from build123d import *

# Parameters (mm, degrees)
SKETCH_1_R          = 21
EXTRUDE_1_DEPTH     = 67
SKETCH_3_R          = 7.5
EXTRUDE_3_DEPTH     = 4.5
SKETCH_4_R          = 2.5
EXTRUDE_4_DEPTH     = 12.7
FILLET_1_R          = 2
FILLET_2_R          = 1
SKETCH_15_R         = 2
CUT_EXTRUDE_2_DEPTH = 5
SKETCH_18_W         = 4.6
SKETCH_18_H         = 0.6
EXTRUDE_11_DEPTH    = 7
SKETCH_19_R         = 7.6
EXTRUDE_12_DEPTH    = 7
EXTRUDE_START       = -39.2
SKETCH_20_R         = 22.175
SKETCH_20_R_2       = 21
EXTRUDE_13_DEPTH    = 34


with BuildPart() as part:
    # 스케치1 → 보스-돌출1 (new body)
    with BuildSketch(Plane(origin=(0, 0, 0), x_dir=(1, 0, 0), z_dir=(0, 1, 0))):
        with Locations(Location((0, 0, 0), (0, 0, 270))):
            Circle(SKETCH_1_R)
    extrude(amount=EXTRUDE_1_DEPTH)

    # 스케치3 → 보스-돌출3 (add)
    with BuildSketch(Plane(origin=(0, 67, 0), x_dir=(1, 0, 0), z_dir=(0, 1, 0))):
        with Locations(Location((0, 0, 0), (0, 0, 270))):
            Circle(SKETCH_3_R)
    extrude(amount=EXTRUDE_3_DEPTH)

    # 스케치4 → 보스-돌출4 (add)
    with BuildSketch(Plane(origin=(0, 71.5, 0), x_dir=(1, 0, 0), z_dir=(0, 1, 0))):
        with Locations(Location((0, 0, 0), (0, 0, 270))):
            Circle(SKETCH_4_R)
    extrude(amount=EXTRUDE_4_DEPTH)

    # 필렛1
    fillet_1_edges = [part.edges().sort_by_distance(p)[0] for p in [
        (0, 67, -21),
    ]]
    fillet(fillet_1_edges, radius=FILLET_1_R)

    # 필렛2
    fillet_2_edges = [part.edges().sort_by_distance(p)[0] for p in [
        (0, 71.5, -7.5),
    ]]
    fillet(fillet_2_edges, radius=FILLET_2_R)

    # 스케치15 → 컷-돌출2 (cut)
    with BuildSketch(Plane(origin=(0, 67, 0), x_dir=(1, 0, 0), z_dir=(0, 1, 0))):
        with Locations(Location((0, 14.5, 0), (0, 0, 270))):
            Circle(SKETCH_15_R)
        with Locations(Location((0, -14.5, 0), (0, 0, 270))):
            Circle(SKETCH_15_R)
    extrude(amount=-CUT_EXTRUDE_2_DEPTH, mode=Mode.SUBTRACT)

    # 스케치18 → 보스-돌출11 (add)
    with BuildSketch(Plane.XZ):
        with Locations((0, 16.35)):
            Rectangle(SKETCH_18_W, SKETCH_18_H)
        with Locations((0, -16.35)):
            Rectangle(SKETCH_18_W, SKETCH_18_H)
    extrude(amount=EXTRUDE_11_DEPTH)

    # 스케치19 → 보스-돌출12 (add)
    with BuildSketch(Plane.XZ):
        with Locations(Location((0, 0, 0), (0, 0, 90))):
            Circle(SKETCH_19_R)
    extrude(amount=EXTRUDE_12_DEPTH)

    # 스케치20 → 보스-돌출13 (add)
    with BuildSketch(Plane(origin=(0, 67, 0), x_dir=(1, 0, 0), z_dir=(0, 1, 0)).offset(EXTRUDE_START)):
        with Locations(Location((0, 0, 0), (0, 0, 270))):
            Circle(SKETCH_20_R)
        with Locations(Location((0, 0, 0), (0, 0, 270))):
            Circle(SKETCH_20_R_2, mode=Mode.SUBTRACT)
    extrude(amount=EXTRUDE_13_DEPTH)


solid = part.part
Build history of the part. All positions in model axes, mm. A direction names the side the tool comes from. Coordinates: 2 decimals unless noted, no trailing zeros. Order: outer loops, then holes, each group sorted by start corner. A loop starts at its lowest first (then second) coordinate and runs counter-clockwise, first axis right, second up. Notation, with made-up numbers: (45, -34) - (63, -34) arc R18 ccw to (63, -22) - close; hole circle Ø1 at (-38, 19.5). An arc over 180 degrees is marked (long way). Write item = value, one per line. Start each with the question number.
1) Saw through at C-C on y = 78. Write the cut outline in (x, z).
2) Saw through at B-B on y = 31.5. Write the cut outline in (x, z) (3 decimals), then the cut area to 3 significant figures.
3) Saw through at A-A on z = 0. Write the cut outline in (x, y) (3 decimals), then the cut area to 3 significant figures.
4) Wall check: line 1 along Y through (x, z) = (8, 3.5); line 2 along X through (y, z) = (12, 0); line 3 along X through (y, z) = (65.5, 14.5). Give the ranges that are in metal, low to high. Write a range as from..to.
5) Flat gauge pins, fed straight in: pin 1 Ø10.5 at (x, z) = (-2.5, -0.5) entering from +Y; pin 2 Ø5 at (x, y) = (-4, 28.5) entering from +Z; pin 3 Ø1.2 at (x, z) = (0, -15) entering from +Y; pin 4 Ø5 at (x, y) = (-1, -4.5) entering from -Z. Where does each tip first touch, or does it go through?
6) 3-axis set-ups, long thin cutter, end or side, ignore diameter. For faces 4 (the face through (0, -3, -16.05)), 5 (the face through (-1.2, 64.5, -16.1)), 6 (the face through (0, -7, 0)), 7 (the face through (0, -3, -16.65)), 8 (the face through (6.31, 13.71, 20.03)): which of +Z, -Z, +X, -X, +Y, -Y reach the whole face in a straight line?
7) Two-plate mould, pull along Z, no slides. Class faces 1 (the face through (0.33, 68.726, -7.493)), 2 (the face through (2.91, -3.45, 7.02)), 3 (the face through (-8, 61.8, 20)): pulls with the +Z half, pulls with the -Z half, needs draft (parallel to the pull), parting line crosses it, or undercut.
From the geometry:
q1.outline = circle Ø5 at (0, 0)
q2.outline = circle Ø44.35 at (0, 0)
q2.area = 1,540 mm^2
q3.outline = (-22.175, 27.8) - (-21, 27.8) - (-21, 0) - (-7.6, 0) - (-7.6, -7) - (7.6, -7) - (7.6, 0) - (21, 0) - (21, 27.8) - (22.175, 27.8) - (22.175, 61.8) - (21, 61.8) - (21, 65) arc R2 ccw to (19, 67) - (7.5, 67) - (7.5, 70.5) arc R1 ccw to (6.5, 71.5) - (2.5, 71.5) - (2.5, 84.2) - (-2.5, 84.2) - (-2.5, 71.5) - (-6.5, 71.5) arc R1 ccw to (-7.5, 70.5) - (-7.5, 67) - (-19, 67) arc R2 ccw to (-21, 65) - (-21, 61.8) - (-22.175, 61.8) - close
q3.area = 3,130 mm^2
q4.line_1 = 0..67
q4.line_2 = -21..21
q4.line_3 = -15.1..-2, 2..15.1
q5.pin_1 = 84.2
q5.pin_2 = 22.12
q5.pin_3 = 62
q5.pin_4 = -16.65
q6.face_4 = +X, -X, -Y
q6.face_5 = +Y
q6.face_6 = +Z, -Z, +X, -X, -Y
q6.face_7 = -Z, +X, -X, -Y
q6.face_8 = -Y
q7.face_1 = parting line crosses it
q7.face_2 = undercut
q7.face_3 = needs draft
